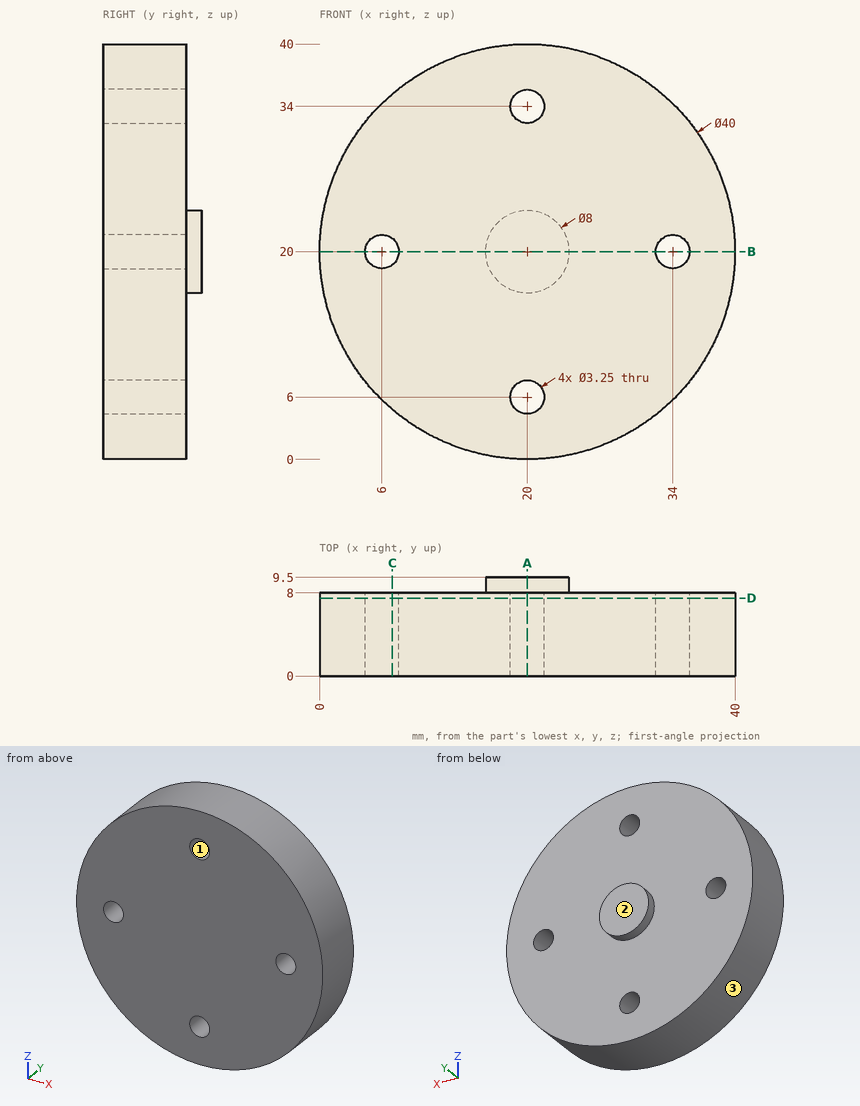
Geometry check sheet. Reference: drawing and pictorial views, mm from the part's lowest x, y, z. Give positions to 0.01 mm unless a question says otherwise; leave off trailing zeros. Order: outer loops, then holes, each group sorted by start corner. A loop starts at its lowest first (then second) coordinate and runs counter-clockwise, first axis right, second up.
1. Section check D-D, the plane y = 7.5. Enter the section's corners in (x, z) (3 decimals), and give its area (3 significant figures).
2. Section check C-C, the plane x = 7. Enter the section's corners in (y, z), and give its area (3 significant figures).
3. Gauge pin test, flat ends, axial feed: pin 1 Ø4 at (x, y) = (19.5, 6.5) entering from +Z; pin 2 Ø3 at (x, z) = (5.5, 33) entering from +Y; pin 3 Ø2 at (x, y) = (33, 2) entering from +Z; pin 4 Ø5 at (y, z) = (4, 33.5) entering from -X. Record the tip position at first contact, or that the pin passes through.
4. Section check B-B, the plane z = 20. Enter the section's corners in (x, y) (3 decimals).
5. Thickness scan on L1, parallel to X at y = 4.25, z = 20 (3 decimals); L2, parallel to Y at x = 26, z = 32; L3, parallel to X at y = 5.5, z = 6 (3 decimals). Record the ranges inside material, lowest first.
6. Section check A-A, the plane x = 20. Enter the section's corners in (y, z) (3 decimals).
7. Release check for a two-part mould opening along X. For the marked faces 1, 2 and 3 record: pulls with the +X half, pulls with the -X half, needs draft (parallel to the pull), parting line crosses it, or undercut.
Values follow:
1. outline: circle Ø40 at (20, 20); hole circle Ø3.25 at (6, 20); hole circle Ø3.25 at (20, 6); hole circle Ø3.25 at (20, 34); hole circle Ø3.25 at (34, 20)
1. area: 1,220 mm2
2. outline: (0, 4.8) - (8, 4.8) - (8, 18.72) - (0, 18.72) - close; (0, 21.28) - (8, 21.28) - (8, 35.2) - (0, 35.2) - close
2. area: 223 mm2
3. pin 1: stops at z = 40
3. pin 2: stops at y = 8
3. pin 3: stops at z = 36
3. pin 4: stops at x = 3.3
4. outline: (0, 0) - (4.375, 0) - (4.375, 8) - (0, 8) - close; (7.625, 0) - (32.375, 0) - (32.375, 8) - (24, 8) - (24, 9.5) - (16, 9.5) - (16, 8) - (7.625, 8) - close; (35.625, 0) - (40, 0) - (40, 8) - (35.625, 8) - close
5. L1: x = 0 to 4.375, 7.625 to 32.375, 35.625 to 40
5. L2: y = 0 to 8
5. L3: x = 5.717 to 18.375, 21.625 to 34.283
6. outline: (0, 0) - (8, 0) - (8, 4.375) - (0, 4.375) - close; (0, 7.625) - (8, 7.625) - (8, 16) - (9.5, 16) - (9.5, 24) - (8, 24) - (8, 32.375) - (0, 32.375) - close; (0, 35.625) - (8, 35.625) - (8, 40) - (0, 40) - close
7. face 1: undercut
7. face 2: needs draft
7. face 3: parting line crosses it
